Work out the finished part from the listing and answer in its coordinate system (mm). A direction names the side the tool comes from. Round coordinates to 2 decimals unless told otherwise and drop trailing zeros. Write each loop counter-clockwise with the first axis right and the second up, starting at its lowest first coordinate (ties: lowest second). Pieces come first, ordered by that corner, then holes. Notation, with made-up numbers: (-31.75, 72.25) - (12.25, 72.25) arc R16 cw to (12.25, 92.25) - close; hole circle Ø7 at (-17, -36.5). An arc over 180 degrees is marked (long way). Answer as a JSON object with one key per item and string values.
Autodesk Inventor part; units mm, degrees
ref_plane "YZ Plane" through (0, 0, 0) normal (1, 0, 0) x (0, 1, 0)
ref_plane "XZ Plane" through (0, 0, 0) normal (0, 1, 0) x (-1, 0, 0)
ref_plane "XY Plane" through (0, 0, 0) normal (0, 0, 1) x (1, 0, 0)
sketch "Sketch1" plane through (0, 0, 0) normal (0, 1, 0) x (-1, 0, 0)
  line L0 (0, 63.5) -> (0, -63.5) construction
  line L1 (-25.4, 63.5) -> (-25.4, -63.5)
  line L2 (25.4, -63.5) -> (25.4, 63.5)
  arc A0 (25.4, 63.5) -> (-25.4, 63.5) centre (0, 63.5) ccw
  arc A1 (-25.4, -63.5) -> (25.4, -63.5) centre (0, -63.5) ccw
  circle A2 centre (0, 63.5) radius 6.35
  circle A3 centre (0, -63.5) radius 6.35
  point P0 (0, 0)
  dimension "d0" = 127
  dimension "d1" = 25.4
  dimension "d2" = 12.7
extrude "Extrusion1" add sketch "Sketch1" along normal blind 12.7
sketch "Sketch2" plane through (0, 0, 0) normal (1, 0, 0) x (0, 1, 0)
  arc A0 (0, -44.45) -> (0, 44.45) centre (0, 0) ccw
  line L0 (0, 44.45) -> (0, -44.45)
  line L1 (0, 63.5) -> (0, -63.5)
  dimension "d5" = 44.45
extrude "Extrusion2" add sketch "Sketch2" along normal mid plane 63.5
sketch "Sketch3" plane through (31.75, 0, 0) normal (1, 0, 0) x (0, 0, -1)
  line L0 (-25.4, 0) -> (25.4, 0)
  line L1 (25.4, 0) -> (25.4, 19.05)
  line L2 (25.4, 19.05) -> (-25.4, 19.05)
  line L3 (-25.4, 19.05) -> (-25.4, 0)
  point P0 (0, 0)
  point P1 (0, 19.05)
  point P2 (0, 0)
  dimension "d8" = 50.8
  dimension "d9" = 19.05
extrude "rectCut" [suppressed]
sketch "Sketch4" plane through (31.75, 0, -25.4) normal (0, -1, 0) x (1, 0, 0)
  circle A0 centre (-31.75, 25.4) radius 1.5875
  dimension "d12" = 3.175
extrude ".125Hole" cut sketch "Sketch4" against normal through all
sketch "Sketch5" plane through (31.75, 0, 0) normal (1, 0, 0) x (0, 0, -1)
  arc A0 (31.75, 0) -> (-31.75, 0) centre (0, 0) ccw
  line L0 (31.75, 0) -> (-31.75, 0)
  dimension "d15" = 31.75
extrude "circCut" [suppressed]
properties part number "ch7-parent"
Item 1: For faces 4 (the flat face through (0, 12.7, -71)), 5 (the cylindrical face through (-0.559, 6.261, -88.894)), determine the directions among +Z, -Z, +X, -X, +Y, -Y from which every point of the face is accessible in a straight line to the end or side of a thin tool.
Results found:
{"face 4": "-Z, +X, -X, +Y", "face 5": "-Z, +Y, -Y"}
Item 2: Consider line 1 along Z through (x, y) = (0, 9); line 2 along X through (y, z) = (5, 63); line 3 along X through (y, z) = (11.5, 0). Determine where each line is inside the solid, lowest interval first.
Results found:
{"line 1": "-88.9 to -69.85, -57.15 to -1.59, 1.59 to 57.15, 69.85 to 88.9", "line 2": "-25.4 to -6.33, 6.33 to 25.4", "line 3": "-31.75 to -1.59, 1.59 to 31.75"}
Item 3: Determine the mould class of faces 1 (the flat face through (31.75, 17, 1)), 2 (the flat face through (6, 12.7, 66)), 3 (the cylindrical face through (1.38, 6.26, -57.3)) for opening direction X: pulls with the +X half, pulls with the -X half, needs draft (parallel to the pull), parting line crosses it, or undercut.
Results found:
{"face 1": "pulls with the +X half", "face 2": "needs draft", "face 3": "undercut"}
Item 4: Each of these flat-tipped pins is pushed along its axis until it touches: P1, Ø6, axis at x = -18, y = 21.5, coming from the -Z side; P2, Ø6.5, axis at y = 8, z = 57.5, coming from the -X side; P3, Ø14, axis at y = 3, z = 51.5, coming from the +X side; P4, Ø7.5, axis at x = 0, z = 63.5, coming from the +Y side. Where does it stop, or does it pass through?
Results found:
{"P1": "z = -40.42", "P2": "x = -25.4", "P3": "x = 25.4", "P4": "through"}
Item 5: A cutting plane is placed at D-D (x = 9). Write down the section's boundary in (y, z), and give its area (3 significant figures).
Results found:
{"outline": "(0, -87.25) - (12.7, -87.25) - (12.7, -42.6) arc R44.45 ccw to (12.7, 42.6) - (12.7, 87.25) - (0, 87.25) - close", "area": "4,210 mm²"}
Item 6: A cutting plane is placed at B-B (x = 0). Write down the section's boundary in (y, z), and give its area (3 significant figures).
Results found:
{"outline": "(0, -88.9) - (12.7, -88.9) - (12.7, -69.85) - (0, -69.85) - close; (0, -57.15) - (12.7, -57.15) - (12.7, -42.6) arc R44.45 ccw to (44.42, -1.59) - (0, -1.59) - close; (0, 1.59) - (44.42, 1.59) arc R44.45 ccw to (12.7, 42.6) - (12.7, 57.15) - (0, 57.15) - close; (0, 69.85) - (12.7, 69.85) - (12.7, 88.9) - (0, 88.9) - close", "area": "3,780 mm²"}
Item 7: A cutting plane is placed at A-A (z = 0). Write down the section's boundary in (x, y).
Results found:
{"outline": "(-31.75, 0) - (-1.59, 0) - (-1.59, 44.45) - (-31.75, 44.45) - close; (1.59, 0) - (31.75, 0) - (31.75, 44.45) - (1.59, 44.45) - close"}
